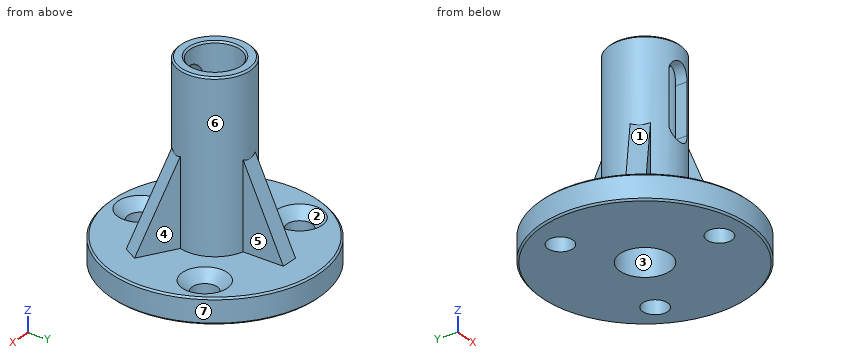
from build123d import *

# Parameters (mm, degrees)
SKETCH1_R               = 12.5
BOSS_EXTRUDE1_DEPTH     = 3
SKETCH2_R               = 4.25
SKETCH2_R_2             = 3
BOSS_EXTRUDE2_DEPTH     = 20
CUT_EXTRUDE2_REACH      = 28.693
SKETCH7_R               = 1.5
CHAMFER3_SIZE           = 1.2
CUT_EXTRUDE4_REACH      = 33.078
CUT_EXTRUDE4_END_RADIUS = 3
CUT_EXTRUDE5_REACH      = 28.693
SKETCH10_R              = 3
RIB3_REACH              = 31.009
SKETCH13_WALL_W         = 71.088033888
SKETCH13_WALL_H         = 2
CIRPATTERN3_COUNT       = 3
CHAMFER8_SIZE           = 0.2


with BuildPart() as part:
    # Sketch1 → Boss-Extrude1 (new body)
    with BuildSketch(Plane.XY):
        Circle(SKETCH1_R)
    extrude(amount=BOSS_EXTRUDE1_DEPTH)

    # Sketch2 → Boss-Extrude2 (add)
    with BuildSketch(Plane.XY.offset(3)):
        Circle(SKETCH2_R)
        Circle(SKETCH2_R_2, mode=Mode.SUBTRACT)
    extrude(amount=BOSS_EXTRUDE2_DEPTH)

    # Sketch7 → Cut-Extrude2 (cut, up to next)
    with BuildSketch(Plane.XY.offset(3), mode=Mode.PRIVATE) as cut_extrude2_sk1:
        with Locations((7.794228634, 4.5)):
            Circle(SKETCH7_R)
    cut_extrude2_tool1 = extrude(cut_extrude2_sk1.sketch, amount=-CUT_EXTRUDE2_REACH, mode=Mode.PRIVATE) & part.part
    # Sketch7 → Cut-Extrude2 (cut, up to next)
    with BuildSketch(Plane.XY.offset(3), mode=Mode.PRIVATE) as cut_extrude2_sk2:
        with Locations((0, -9)):
            Circle(SKETCH7_R)
    cut_extrude2_tool2 = extrude(cut_extrude2_sk2.sketch, amount=-CUT_EXTRUDE2_REACH, mode=Mode.PRIVATE) & part.part
    # Sketch7 → Cut-Extrude2 (cut, up to next)
    with BuildSketch(Plane.XY.offset(3), mode=Mode.PRIVATE) as cut_extrude2_sk3:
        with Locations((-7.794228634, 4.5)):
            Circle(SKETCH7_R)
    cut_extrude2_tool3 = extrude(cut_extrude2_sk3.sketch, amount=-CUT_EXTRUDE2_REACH, mode=Mode.PRIVATE) & part.part
    add(cut_extrude2_tool1.solids().sort_by_distance((7.794229, 4.5, 3))[0], mode=Mode.SUBTRACT)
    add(cut_extrude2_tool2.solids().sort_by_distance((0, -9, 3))[0], mode=Mode.SUBTRACT)
    add(cut_extrude2_tool3.solids().sort_by_distance((-7.794229, 4.5, 3))[0], mode=Mode.SUBTRACT)

    # Chamfer3
    chamfer3_edges = [part.edges().sort_by_distance(p)[0] for p in [
        (6.294228634, 4.5, 3),
        (-1.5, -9, 3),
        (-9.294228634, 4.5, 3),
    ]]
    chamfer(chamfer3_edges, length=CHAMFER3_SIZE)

    # Cut-Extrude4: up to this cylinder (the profile starts outside it)
    cut_extrude4_end = Plane(origin=(0, 0, 16.5), z_dir=(0, 0, -1)) * Cylinder(CUT_EXTRUDE4_END_RADIUS, 73.156, mode=Mode.PRIVATE)
    # Sketch9 → Cut-Extrude4 (cut, up to the surface)
    with BuildSketch(Plane(origin=(0, -4.25, 0), x_dir=(1, 0, 0), z_dir=(0, 1, 0)), mode=Mode.PRIVATE) as cut_extrude4_sk1:
        with BuildLine():
            Line((-1.5, -13.5), (-1.5, -19.5))
            ThreePointArc((-1.5, -19.5), (0, -21), (1.5, -19.5))
            Line((1.5, -19.5), (1.5, -13.5))
            ThreePointArc((1.5, -13.5), (0, -12), (-1.5, -13.5))
        make_face()
    cut_extrude4_tool1 = extrude(cut_extrude4_sk1.sketch, amount=CUT_EXTRUDE4_REACH, mode=Mode.PRIVATE) - cut_extrude4_end
    add(cut_extrude4_tool1.solids().sort_by_distance((0, -4.25, 16.5))[0], mode=Mode.SUBTRACT)

    # Sketch10 → Cut-Extrude5 (cut, up to next)
    with BuildSketch(Plane.XY.offset(3), mode=Mode.PRIVATE) as cut_extrude5_sk1:
        Circle(SKETCH10_R)
    cut_extrude5_tool1 = extrude(cut_extrude5_sk1.sketch, amount=-CUT_EXTRUDE5_REACH, mode=Mode.PRIVATE) & part.part
    add(cut_extrude5_tool1.solids().sort_by_distance((0, 0, 3))[0], mode=Mode.SUBTRACT)

    # Sketch13 wall → Rib3 (add, up to next)
    with BuildSketch(Plane(origin=(0, 6.625, 8), x_dir=(0, -0.429056814568, 0.903277504354), z_dir=(0, -0.903277504354, -0.429056814568)), mode=Mode.PRIVATE) as rib3_sk1:
        Rectangle(SKETCH13_WALL_W, SKETCH13_WALL_H)
    rib3_tool1 = extrude(rib3_sk1.sketch, amount=RIB3_REACH, mode=Mode.PRIVATE) - part.part
    rib3 = rib3_tool1.solids().sort_by_distance((0, 6.625, 8))[0]
    add(rib3)

    # CirPattern3: Rib3 ×3 about axis
    cirpattern3_axis = Axis((0, 0, 0), (0, 0, 1))
    for i in range(1, CIRPATTERN3_COUNT):
        add(rib3.rotate(cirpattern3_axis, i * 360 / CIRPATTERN3_COUNT))

    # Chamfer8
    chamfer8_edges = [part.edges().sort_by_distance(p)[0] for p in [
        (-12.5, 0, 0),
        (-12.5, 0, 3),
        (-4.25, 0, 23),
        (-3, 0, 23),
    ]]
    chamfer(chamfer8_edges, length=CHAMFER8_SIZE)


solid = part.part
Verification items for the finished model (mm, model axes). Face numbers are marked on the shaded views. A direction names the side the tool comes from. Give positions to 0.01 mm unless a question says otherwise; leave off trailing zeros. Order: outer loops, then holes, each group sorted by start corner. A loop starts at its lowest first (then second) coordinate and runs counter-clockwise, first axis right, second up. Notation, with made-up numbers: M -25.75,37 L -19.75,37 A18 cw -19.75,45 Z; hole C 77.25,69.25 d6. An arc over 180 degrees is marked long. Use one line per item in the form item = value. Start each with the question number.
Q1. Section check B-B (x = 0). Count the separate pieces of the cut face and the enclosed holes in it, then the cut area to 3 significant figures.
Q2. Section check D-D (z = 15.75). Enter the section's corners in (x, y), then the cut area to 3 significant figures.
Q3. Access from +Z, -Z, +X, -X, +Y, -Y to the whole of each face (thin tool, end or side, straight path). Record for the marked faces 5, 6 and 7.
Q4. Section check C-C (z = 8.75). Enter the section's corners in (x, y), then the cut area to 3 significant figures.
Q5. Scan lines: line 1 along Y through (x, z) = (0, 0.55); line 2 along Z through (x, y) = (-5.5, -8.75); line 3 along X through (y, z) = (-2.75, 9.5). Record each from-to range of solid material in increasing order. Write a range as [from, to].
Q6. Mould release check, pull along X, two halves, no side actions. Record for the marked faces 1, 2, 3 and 4: +X half, -X half, draft (parallel to the pull), parting line (faces both ways), or undercut.
Q7. Go/stop test with flat-tipped pins: pin 1 Ø5 at (y, z) = (6, 3.5) entering from -X; pin 2 Ø1.5 at (x, z) = (-2, 5) entering from +Y; pin 3 Ø4 at (x, z) = (1.5, 10) entering from -Y. Record where each tip stops, or that it passes through.
Q8. Section check A-A (y = 0). Enter the section's corners in (x, z).
Evaluation:
q1.separate_pieces = 4
q1.enclosed_holes = 0
q1.area = 109 mm2
q2.outline = M -1.5,-3.98 L -1.5,-2.6 A3 cw long 1.5,-2.6 L 1.5,-3.98 A4.25 ccw long Z
q2.area = 24.6 mm2
q3.face_5 = +Z, +X, +Y
q3.face_6 = +Z
q3.face_7 = +Z, -Z
q4.outline = M -5.93,-2.27 L -4.93,-4 L -3.08,-2.93 A4.25 ccw 3.08,-2.93 L 4.93,-4 L 5.93,-2.27 L 4.08,-1.2 A4.25 ccw 1,4.13 L 1,6.27 L -1,6.27 L -1,4.13 A4.25 ccw -4.08,-1.2 Z; hole C 0,0 d6
q4.area = 40.8 mm2
q5.line_1 = [-12.5, -10.5], [-7.5, -3], [3, 12.5]
q5.line_2 = [0, 3]
q5.line_3 = [-5.24, -1.2], [1.2, 5.24]
q6.face_1 = -X half
q6.face_2 = undercut
q6.face_3 = undercut
q6.face_4 = +X half
q7.pin_1 = -11.97
q7.pin_2 = 4.06
q7.pin_3 = -4.25
q8.outline = M -12.5,0.2 L -12.3,0 L -3,0 L -3,22.8 L -3.2,23 L -4.05,23 L -4.25,22.8 L -4.25,3 L -12.3,3 L -12.5,2.8 Z; M 3,0 L 12.3,0 L 12.5,0.2 L 12.5,2.8 L 12.3,3 L 4.25,3 L 4.25,22.8 L 4.05,23 L 3.2,23 L 3,22.8 Z
